Model file for the job. Use its own axes, mm. A direction names the side the tool comes from. Coordinates: 2 decimals unless noted, no trailing zeros. Write each loop counter-clockwise with the first axis right and the second up, starting at its lowest first coordinate (ties: lowest second). Pieces come first, ordered by that corner, then holes.
Q1. Pin check, flat tips, straight feed: P1, Ø1.5, axis at y = -2.5, z = 85, coming from the -X side; P2, Ø10, axis at y = 3, z = 39.5, coming from the -X side (3 decimals); P3, Ø3, axis at x = -3.5, z = 18, coming from the +Y side. Stop position of each tip, or through.
Q2. Drill centre lines: probe 1 along Z at (x, y) = (-5, 10); probe 2 along Y at (x, z) = (-2.75, 83); probe 3 along X at (y, z) = (0, 58) (3 decimals). Where is each one in solid material? Low to high.
Q3. Which spindle directions (+Z, -Z, +X, -X, +Y, -Y) get a long thin tool onto all of the face, cutting with end or side? Do faces 1 (the cylindrical face through (-16, 0, 80)), 2 (the flat face through (-2, -10, 85)), 3 (the flat face through (-3, 0, 85)), 4 (the flat face through (-2, 10, 85)), 5 (the cylindrical face through (-3.084, 0.068, 38.074)). Say none if no direction does.
Q4. Band-saw the part on B-B, the plane x = -10.5. Write the cut outline in (y, z), plus the area to 3 significant figures.
Q5. Band-saw the part on C-C, the plane z = 49. Write the cut outline in (x, y) (3 decimals), plus the area to 3 significant figures.
Q6. Band-saw the part on A-A, the plane y = 0. Write the cut outline in (x, z) (3 decimals).
Q7. Band-saw the part on D-D, the plane y = 6. Write the cut outline in (x, z).
from build123d import *

# Parameters (mm, degrees)
CROQUIS11_R             = 3.085
SALIENTE_EXTRUIR2_DEPTH = 77.23
CROQUIS12_R             = 16
SALIENTE_EXTRUIR3_DEPTH = 5
CROQUIS13_W             = 6
CROQUIS13_H             = 20
SALIENTE_EXTRUIR4_DEPTH = 5
CORTAR_EXTRUIR9_REACH   = 92.117
CROQUIS14_W             = 16
CROQUIS14_H             = 32


with BuildPart() as part:
    # Croquis11 → Saliente-Extruir2 (new body)
    with BuildSketch(Plane.XY):
        Circle(CROQUIS11_R)
    extrude(amount=SALIENTE_EXTRUIR2_DEPTH)

    # Croquis12 → Saliente-Extruir3 (add)
    with BuildSketch(Plane.XY.offset(77.23)):
        Circle(CROQUIS12_R)
    extrude(amount=SALIENTE_EXTRUIR3_DEPTH)

    # Croquis13 → Saliente-Extruir4 (add)
    with BuildSketch(Plane.XY.offset(82.23)):
        Rectangle(CROQUIS13_W, CROQUIS13_H)
    extrude(amount=SALIENTE_EXTRUIR4_DEPTH)

    # Cortar-Extruir9: up to this face of the body (flat: up to its plane)
    cortar_extruir9_end = Plane(part.part.faces().sort_by_distance((0, 0, 0))[0])
    # Croquis14 → Cortar-Extruir9 (cut, up to the picked face)
    with BuildSketch(Plane.XY.offset(87.23), mode=Mode.PRIVATE) as cortar_extruir9_sk1:
        with Locations((8, 0)):
            Rectangle(CROQUIS14_W, CROQUIS14_H)
    cortar_extruir9_tool1 = split(extrude(cortar_extruir9_sk1.sketch, amount=-CORTAR_EXTRUIR9_REACH, mode=Mode.PRIVATE), bisect_by=cortar_extruir9_end, keep=Keep.BOTH, mode=Mode.PRIVATE)
    add(cortar_extruir9_tool1.solids().sort_by(Axis((8, 0, 87.23), (0, 0, -1)))[0], mode=Mode.SUBTRACT)


solid = part.part
Answer sheet:
1. P1: stops at x = -3
1. P2: stops at x = -3.085
1. P3: stops at y = 2.35
2. probe 1: z = 77.23 to 82.23
2. probe 2: y = -10 to 10
2. probe 3: x = -3.085 to 0
3. face 1: +Z, -Z, -X
3. face 2: +Z, +X, -X, -Y
3. face 3: +Z, -X, +Y, -Y
3. face 4: +Z, +X, -X, +Y
3. face 5: -Z, -X
4. outline: (-12.07, 77.23) - (12.07, 77.23) - (12.07, 82.23) - (-12.07, 82.23) - close
4. area: 121 mm2
5. outline: (0, -3.085) - (0, 3.085) arc R3.085 ccw to start
5. area: 14.9 mm2
6. outline: (-16, 77.23) - (-3.085, 77.23) - (-3.085, 0) - (0, 0) - (0, 87.23) - (-3, 87.23) - (-3, 82.23) - (-16, 82.23) - close
7. outline: (-14.83, 77.23) - (0, 77.23) - (0, 87.23) - (-3, 87.23) - (-3, 82.23) - (-14.83, 82.23) - close
